```python
from build123d import *

# Parameters (mm, degrees)
SKETCH_1_W          = 33.5
SKETCH_1_H          = 15
SKETCH_1_R          = 3.624978968
SKETCH_1_R_2        = 3.60228421
EXTRUDE_1_DEPTH     = 2
SKETCH_1_3_W        = 1
SKETCH_1_3_H        = 15
EXTRUDE_2_DEPTH     = 6
SKETCH_2_R          = 1.6
EXTRUDE_3_DEPTH     = 1.5
EXTRUDE_4_DEPTH     = 5
SKETCH_4_W          = 3
SKETCH_4_H          = 5
EXTRUDE_5_DEPTH     = 10
SKETCH_5_R          = 1.6
CUT_EXTRUDE_1_DEPTH = 10


with BuildPart() as part:
    # Sketch 1 → Extrude 1 (new body)
    with BuildSketch(Plane(origin=(0, 0, 0), x_dir=(1, 0, 0), z_dir=(0, 1, 0))):
        Rectangle(SKETCH_1_W, SKETCH_1_H)
        with Locations((-4.032505812, 2.018294601)):
            Circle(SKETCH_1_R, mode=Mode.SUBTRACT)
        with Locations((3.968074022, 2.018294601)):
            Circle(SKETCH_1_R_2, mode=Mode.SUBTRACT)
    extrude(amount=EXTRUDE_1_DEPTH)

    # Sketch 1_3 → Extrude 2 (add)
    with BuildSketch(Plane(origin=(0, 0, 0), x_dir=(1, 0, 0), z_dir=(0, 1, 0))):
        with Locations((-16.25, 0)):
            Rectangle(SKETCH_1_3_W, SKETCH_1_3_H)
        with Locations((16.25, 0)):
            Rectangle(SKETCH_1_3_W, SKETCH_1_3_H)
    extrude(amount=-EXTRUDE_2_DEPTH)

    # Sketch 2 → Extrude 3 (add)
    with BuildSketch(Plane.XZ.offset(6)):
        Polygon((-16.75, -7.5), (-24.597168746, -7.5), (-24.597168746, 0), (-24.597168746, 7.5), (-16.75, 7.5), (-16.75, 0), align=None)
        with Locations((-20.395135673, 2.61052916)):
            Circle(SKETCH_2_R, mode=Mode.SUBTRACT)
        Polygon((16.75, 7.5), (22.842739313, 7.5), (22.842739313, 0), (22.842739313, -7.5), (16.75, -7.5), (16.75, 0), align=None)
        with Locations((19.826698125, 4.651883457)):
            Circle(SKETCH_2_R, mode=Mode.SUBTRACT)
    extrude(amount=-EXTRUDE_3_DEPTH)

    # Sketch 3 → Extrude 4 (add)
    with BuildSketch(Plane(origin=(0, 0, -7.5), x_dir=(-1, 0, 0), z_dir=(0, 0, -1))):
        Polygon((-16.75, 2), (-16.75, -4.5), (-22.842739313, -4.5), (-22.842739313, -6), (-15.75, -6), (-15.75, 0), (15.75, 0), (15.75, -6), (24.597168746, -6), (24.597168746, -4.5), (16.75, -4.5), (16.75, 2), align=None)
    extrude(amount=EXTRUDE_4_DEPTH)

    # Sketch 4 → Extrude 5 (add)
    with BuildSketch(Plane(origin=(0, 2, 0), x_dir=(1, 0, 0), z_dir=(0, 1, 0))):
        with Locations((0, 10)):
            Rectangle(SKETCH_4_W, SKETCH_4_H)
    extrude(amount=EXTRUDE_5_DEPTH)

    # Sketch 5 → Cut-Extrude 1 (cut)
    with BuildSketch(Plane(origin=(1.5, 0, 0), x_dir=(0, 0, -1), z_dir=(1, 0, 0))):
        with Locations((10, 9.5)):
            Circle(SKETCH_5_R)
    extrude(amount=-CUT_EXTRUDE_1_DEPTH, mode=Mode.SUBTRACT)


solid = part.part
```
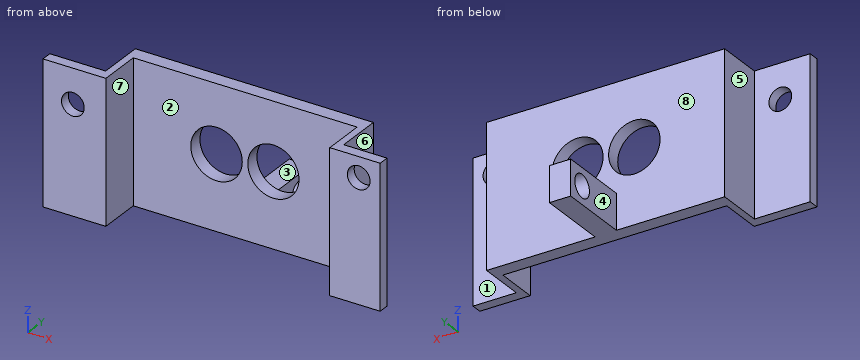
Model file for the job. Use its own axes, mm. Face numbers are marked on the shaded views. A direction names the side the tool comes from. Coordinates: 2 decimals unless noted, no trailing zeros. Order: outer loops, then holes, each group sorted by start corner. A loop starts at its lowest first (then second) coordinate and runs counter-clockwise, first axis right, second up. Notation, with made-up numbers: (78.5, 8) -> (84.5, 8) arc R26 ccw to (84.5, 43) -> close; hole circle Ø2 at (-11.75, -25). An arc over 180 degrees is marked (long way). Answer as a JSON object with one key per item and string values. Group by question number.
1) Flat gauge pins, fed straight in: pin 1 (11.5 mm diameter, centred on x = 3.97, z = -2.02, fed in from +Y); pin 2 (3.5 mm diameter, centred on x = 0.5, y = 8, fed in from +Z); pin 3 (5 mm diameter, centred on x = 8.5, z = -7, fed in from -Y); pin 4 (3 mm diameter, centred on x = -14, y = -3.5, fed in from +Z). Where does each tip first touch, or does it go through?
2) Cut at D-D, the plane y = 9.5. Write the cut outline in (x, z), then the cut area to 3 significant figures.
3) Drill centre lines: L1, parallel to X at y = -4, z = -3; L2, parallel to Z at x = -4.5, y = 1.75; L3, parallel to X at y = 0.5, z = -5. Where is each one in solid material? Low to high.
4) Cut at A-A, the plane y = -3.5. Write the cut outline in (x, z).
5) Pull direction X, two halves, no side cores. Call the marked faces 5, 6, 7 and 8: +X half, -X half, draft (parallel to the pull), parting line (faces both ways), or undercut.
6) Which spindle directions (+Z, -Z, +X, -X, +Y, -Y) get a long thin tool onto all of the face, cutting with end or side? Do the marked faces 1, 2, 3 and 4. Say none if no direction does.
7) Cut at C-C, the plane x = 1. Write the cut outline in (y, z).
8) Cut at B-B, the plane z = -9.5. Write the cut outline in (x, y), then the cut area to 3 significant figures.
Check values:
{
 "1": {"pin 1": "stops at y = 2", "pin 2": "stops at z = -7.5", "pin 3": "stops at y = 0", "pin 4": "passes through"},
 "2": {"outline": "(-1.5, -12.5) -> (1.5, -12.5) -> (1.5, -11.6) -> (-1.5, -11.6) -> close; (-1.5, -8.4) -> (1.5, -8.4) -> (1.5, -7.5) -> (-1.5, -7.5) -> close", "area": "5.40 mm²"},
 "3": {"L1": "x = -16.75 to -15.75, 15.75 to 16.75", "L2": "z = -12.5 to -5.61, 1.58 to 7.5", "L3": "x = -16.75 to -6.09, -1.97 to 1.95, 5.99 to 16.75"},
 "4": {"outline": "(-16.75, -12.5) -> (-15.75, -12.5) -> (-15.75, 7.5) -> (-16.75, 7.5) -> close; (15.75, -12.5) -> (16.75, -12.5) -> (16.75, 7.5) -> (15.75, 7.5) -> close"},
 "5": {"face 5": "-X half", "face 6": "+X half", "face 7": "undercut", "face 8": "draft"},
 "6": {"face 1": "+Z, -Z, +X, +Y", "face 2": "+Z, -Z, -Y", "face 3": "+Z, +X, -X, +Y", "face 4": "+Z, -Z, -X, +Y"},
 "7": {"outline": "(0, -12.5) -> (12, -12.5) -> (12, -7.5) -> (2, -7.5) -> (2, -4.06) -> (0, -4.06) -> close; (0, 0.02) -> (2, 0.02) -> (2, 7.5) -> (0, 7.5) -> close; hole circle Ø3.2 at (9.5, -10)"},
 "8": {"outline": "(-24.6, -6) -> (-15.75, -6) -> (-15.75, 0) -> (15.75, 0) -> (15.75, -6) -> (22.84, -6) -> (22.84, -4.5) -> (16.75, -4.5) -> (16.75, 2) -> (1.5, 2) -> (1.5, 7.98) -> (-1.5, 7.98) -> (-1.5, 2) -> (-16.75, 2) -> (-16.75, -4.5) -> (-24.6, -4.5) -> close; (-1.5, 11.02) -> (1.5, 11.02) -> (1.5, 12) -> (-1.5, 12) -> close", "area": "121 mm²"}
}
